Part model, mm, in its own coordinate system. A direction names the side the tool comes from. Give positions to 0.01 mm unless a question says otherwise; leave off trailing zeros. Order: outer loops, then holes, each group sorted by start corner. A loop starts at its lowest first (then second) coordinate and runs counter-clockwise, first axis right, second up. Notation, with made-up numbers: (-15.5, 9) - (10.5, 9) arc R23 cw to (10.5, 45) - close; hole circle Ø10 at (70, 53). An arc over 180 degrees is marked (long way). One line per item, written item: value.
Autodesk Inventor part; units mm, degrees
ref_plane "Work Plane1" through (-13.5, -13.5, -4) normal (0, 0, 1) x (1, 0, 0)
ref_plane "YZ Plane" through (0, 0, 0) normal (1, 0, 0) x (0, 1, 0)
ref_plane "XZ Plane" through (0, 0, 0) normal (0, 1, 0) x (-1, 0, 0)
sketch "Sketch1" plane through (0, 0, 0) normal (0, 0, 1) x (1, 0, 0)
  line L0 (16.8, 24.9006) -> (-16.8, 24.9006)
  line L1 (-16.8, 24.9006) -> (-16.8, 21.2406)
  line L2 (-16.8, 21.2406) -> (-21.2406, 16.8)
  line L3 (-21.2406, 16.8) -> (-24.9006, 16.8)
  line L4 (-24.9006, 16.8) -> (-24.9006, -16.8)
  line L5 (-24.9006, -16.8) -> (-21.2406, -16.8)
  line L6 (-21.2406, -16.8) -> (-16.8, -21.2406)
  line L7 (-16.8, -21.2406) -> (-16.8, -24.9006)
  line L8 (-16.8, -24.9006) -> (16.8, -24.9006)
  line L9 (16.8, -24.9006) -> (16.8, -21.2406)
  line L10 (16.8, -21.2406) -> (21.2406, -16.8)
  line L11 (21.2406, -16.8) -> (24.9006, -16.8)
  line L12 (24.9006, -16.8) -> (24.9006, 16.8)
  line L13 (24.9006, 16.8) -> (21.2406, 16.8)
  line L14 (21.2406, 16.8) -> (16.8, 21.2406)
  line L15 (16.8, 21.2406) -> (16.8, 24.9006)
  arc A0 (-24.9006, -4.1858) -> (-4.1858, -24.9006) centre (0, 0) ccw
  circle A1 centre (0, 0) radius 19.1
  circle A2 centre (0, 0) radius 18.1
  circle A3 centre (0, 0) radius 20.6
  circle A4 centre (0, 0) radius 19.6 construction
  circle A5 centre (0, 0) radius 20.6 construction
  circle A6 centre (0, 0) radius 20.6 construction
  point P0 (0, 0)
  dimension "d14" = 38.2
  dimension "d17" = 1
ref_plane "Work Plane1" through (-13.5, -13.5, -4) normal (0, 0, 1) x (1, 0, 0)
extrude "Extrusion1" add sketch "Sketch1" against normal blind 4 draft -2 contours A1
sketch "Sketch2" plane through (0, 0, 0) normal (0, 0, 1) x (1, 0, 0)
  line L0 (0, -33.742) -> (0, 37.252) construction
  arc A0 (2, 25.1004) -> (-2, 25.1004) centre (0, 25.11) ccw
  circle A1 centre (0, 0) radius 19.1
  circle A2 centre (0, 0) radius 21.1
  circle A3 centre (0, 0) radius 18.2397
  point P0 (0, 0)
  dimension "d5" = 2
  dimension "d16" = 2
extrude "Extrusion2" add sketch "Sketch2" along normal blind 1 contours A1 | A2
properties part number "20_Lens_holder_156mm_clamp"
1) Which spindle directions (+Z, -Z, +X, -X, +Y, -Y) get a long thin tool onto all of the face, cutting with end or side? Do faces 1 (the flat face through (-11, 16, 0)), 2 (the cylindrical face through (20.126, -6.338, 0.493)), 3 (the cylindrical face through (-3.954, 17.806, 0.493)). Say none if no direction does.
Outcome:
face 1: -Z
face 2: +Z, -Z
face 3: +Z
2) Cut at A-A, the plane x = 0. Give the cut face in (y, z).
Outcome:
outline: (-21.1, 0) - (-19.1, 0) - (-18.96, -4) - (-18.24, -4) - (-18.1, 0) - (-18.24, 0) - (-18.24, 1) - (-21.1, 1) - close; (18.1, 0) - (18.24, -4) - (18.96, -4) - (19.1, 0) - (21.1, 0) - (21.1, 1) - (18.24, 1) - (18.24, 0) - close
3) Drill centre lines: line 1 along Y through (x, z) = (0, 0.2); line 2 along Y through (x, z) = (8, -2.4); line 3 along X through (y, z) = (-1.5, -2.5). Where is each one in solid material? Low to high. Write a range as from..to.
Outcome:
line 1: y = -21.1..-18.24, 18.24..21.1
line 2: y = -17.25..-16.33, 16.33..17.25
line 3: x = -18.95..-18.13, 18.13..18.95
4) Pin check, flat tips, straight feed: pin 1 (1.5 mm diameter, centred on y = -7.5, z = -1.5, fed in from +X); pin 2 (4 mm diameter, centred on x = -4.5, y = -14, fed in from -Z); pin 3 (1 mm diameter, centred on y = -5, z = 0, fed in from +X); pin 4 (1.5 mm diameter, centred on x = 2, z = -2.5, fed in from +Y). Stop position of each tip, or through.
Outcome:
pin 1: stops at x = 17.81
pin 2: passes through
pin 3: stops at x = 20.61
pin 4: stops at y = 18.98
